Autodesk Inventor part; units mm, degrees
ref_plane "YZ Plane" through (0, 0, 0) normal (1, 0, 0) x (0, 1, 0)
ref_plane "XZ Plane" through (0, 0, 0) normal (0, 1, 0) x (-1, 0, 0)
ref_plane "XY Plane" through (0, 0, 0) normal (0, 0, 1) x (1, 0, 0)
sketch "Esboço9" plane through (0, 0, 0) normal (0, 0, 1) x (1, 0, 0)
  line L0 (-215, -43.375) -> (215, -43.375)
  line L1 (215, -43.375) -> (215, 42.625)
  line L2 (215, 42.625) -> (214.25, 42.625)
  line L3 (214.25, 42.625) -> (214.25, -42.625)
  line L4 (214.25, -42.625) -> (-214.25, -42.625)
  line L5 (-214.25, -42.625) -> (-214.25, 42.625)
  line L6 (-214.25, 42.625) -> (-215, 42.625)
  line L7 (-215, 42.625) -> (-215, -43.375)
  point P0 (0, 0)
  dimension "d60" = 430
  dimension "d61" = 86
  dimension "d64" = 85.25
  dimension "d65" = 428.5
  dimension "d67" = 0.75
  dimension "d107" = 214.25
  dimension "d109" = 42.625
extrude "Extrusão6" add sketch "Esboço9" against normal blind 180
sketch "Esboço10" plane through (-214.25, -42.625, 0) normal (0, 1, 0) x (1, 0, 0)
  line L0 (428.5, 0) -> (0, 0)
  line L1 (428.5, 0) -> (428.5, 0.75)
  line L2 (428.5, 0) -> (428.5, 180)
  line L3 (428.5, 0.75) -> (0, 0.75)
  line L4 (0, 0) -> (0, 180)
  line L5 (0, 180) -> (428.5, 180)
  line L6 (0, 180) -> (0, 179.25)
  line L7 (0, 0) -> (0, 180)
  line L8 (0, 179.25) -> (428.5, 179.25)
  line L9 (428.5, 179.25) -> (428.5, 180)
  line L10 (429.25, 180) -> (-0.75, 180)
  line L11 (0, 0.75) -> (0, 0)
  line L12 (-0.75, 0) -> (429.25, 0)
  line L13 (0, 180) -> (428.5, 180)
  point P0 (214.25, 0)
  dimension "d95" = 0.75
  dimension "d96" = 0.75
extrude "Extrusão7" add sketch "Esboço10" along normal blind 4.25 contours L0 L4 L3 L1 | L8 L4 L5 L2
sketch "Esboço11" plane through (214.25, 42.625, -180) normal (-1, 0, 0) x (0, 0, 1)
  line L0 (0, -81) -> (0.75, -81)
  line L1 (0.75, -81) -> (0, -81)
  line L2 (180, 0) -> (0, 0)
  line L3 (0, -81) -> (0, 0)
  line L4 (180, 0) -> (180, -81)
  line L5 (0, 0) -> (180, 0)
  line L6 (180, 0) -> (180, -81)
  line L7 (179.25, -81) -> (180, -81)
  line L8 (180, -81) -> (179.25, -81)
  line L9 (179.25, -81) -> (179.25, -0.75)
  line L10 (179.25, -0.75) -> (0.75, -0.75)
  line L11 (0.75, -0.75) -> (0.75, -81)
  point P0 (180, -42.625)
  dimension "d100" = 178.5
  dimension "d110" = 81
  dimension "d111" = 80.25
extrude "Extrusão8" add sketch "Esboço11" along normal blind 4.25
sketch "Esboço12" plane through (-214.25, 42.625, 0) normal (1, 0, 0) x (0, 0, -1)
  line L0 (0, -81) -> (0.75, -81)
  line L1 (0.75, -81) -> (0, -81)
  line L2 (0, -81) -> (0, 0)
  line L3 (180, -86) -> (180, 0)
  line L4 (0, 0) -> (180, 0)
  line L5 (179.25, -81) -> (180, -81)
  line L6 (180, 0) -> (180, -81)
  line L7 (180, -81) -> (179.25, -81)
  line L8 (179.25, -81) -> (179.25, -0.75)
  line L9 (179.25, -0.75) -> (0.75, -0.75)
  line L10 (0, -81) -> (0, 0)
  line L11 (0.75, -0.75) -> (0.75, -81)
  point P0 (0, -42.625)
  dimension "d103" = 80.25
  dimension "d104" = 178.5
  dimension "d112" = 81
extrude "Extrusão9" add sketch "Esboço12" along normal blind 4.25
sketch "Esboço15" plane through (-214.25, -42.625, -0.75) normal (0, 1, 0) x (1, 0, 0)
  circle A0 centre (311.2625, 145.825) radius 1.75
  circle A1 centre (288.7625, 89.075) radius 1.75
  line L0 (0, 0) -> (428.5, 0)
  line L1 (428.5, 0) -> (428.5, 178.5)
  line L2 (428.5, 178.5) -> (0, 178.5)
  line L3 (0, 0) -> (0, 178.5)
  circle A2 centre (260.7625, 89.075) radius 1.75
  circle A3 centre (238.2625, 145.825) radius 1.75
  circle A4 centre (192.2625, 145.825) radius 1.75
  circle A5 centre (169.7625, 89.075) radius 1.75
  circle A6 centre (141.7625, 89.075) radius 1.75
  circle A7 centre (119.2625, 145.825) radius 1.75
  circle A8 centre (91.2625, 145.825) radius 1.75
  circle A9 centre (68.7625, 89.075) radius 1.75
  circle A10 centre (40.7625, 89.075) radius 1.75
  circle A11 centre (18.2625, 145.825) radius 1.75
  circle A12 centre (339.2625, 145.825) radius 1.75
  circle A13 centre (389.7875, 89.3) radius 1.75
  circle A14 centre (412.2625, 145.825) radius 1.75
  circle A15 centre (361.7875, 89.3) radius 1.75
  point P0 (214.25, -0.75)
hole "Furo5" at (-195.9875, -42.625, -146.575) at (-122.9875, -42.625, -146.575) at (-145.4875, -42.625, -89.825) at (-173.4875, -42.625, -89.825) at (-94.9875, -42.625, -146.575) at (-72.4875, -42.625, -89.825) at (-44.4875, -42.625, -89.825) at (-21.9875, -42.625, -146.575) at (24.0125, -42.625, -146.575) at (46.5125, -42.625, -89.825) at (74.5125, -42.625, -89.825) at (97.0125, -42.625, -146.575) at (125.0125, -42.625, -146.575) at (198.0125, -42.625, -146.575) at (175.5375, -42.625, -90.05) at (147.5375, -42.625, -90.05) direction (0, -1, 0) diameter 2.459 end through all
properties part number "Ra-Manager_Base"
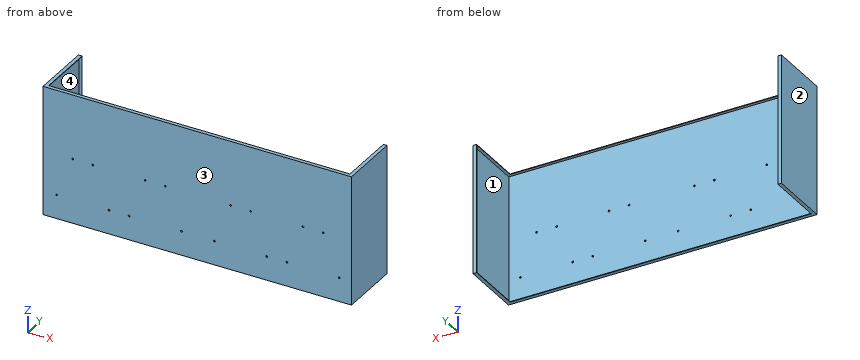
Work out the finished part from the listing and answer in its coordinate system (mm). Face numbers are marked on the shaded views. A direction names the side the tool comes from. Give positions to 0.01 mm unless a question says otherwise; leave off trailing zeros. Write each loop counter-clockwise with the first axis right and the second up, starting at its lowest first coordinate (ties: lowest second). Pieces come first, ordered by that corner, then holes.
(1) The mould has two halves that part along Z. Classify the marked faces 3 and 4: pulls with the +Z half, pulls with the -Z half, needs draft (parallel to the pull), parting line crosses it, or undercut.
Final values:
face 3: needs draft
face 4: undercut
(2) A flat-ended cylindrical pin translates along its axis: pin 1 Ø2 at (x, z) = (-10.5, -56.5) entering from +Y (3 decimals). Find the tip coordinate at first contact, or state that the pin passes through.
Final values:
pin 1: stops at y = -42.625
(3) The part is cut by section A-A on z = -47.5. Write down the section's boundary in (x, y) (3 decimals), plus the area to 3 significant figures.
Final values:
outline: (-215, -43.375) - (215, -43.375) - (215, 42.625) - (210, 42.625) - (210, 41.875) - (214.25, 41.875) - (214.25, -42.625) - (-214.25, -42.625) - (-214.25, 41.875) - (-210, 41.875) - (-210, 42.625) - (-215, 42.625) - close
area: 457 mm2
(4) Straight lines are drawn through the part: line 1 (X direction, y = 9.5, z = -108.5); line 2 (Y direction, x = 31, z = -51) (3 decimals). For each, find the intervals that lie inside material, in ascending order.
Final values:
line 1: x = -215 to -214.25, 214.25 to 215
line 2: y = -43.375 to -42.625
(5) Which of the six approach directions +Z, -Z, +X, -X, +Y, -Y give full straight-line access (tool end or side, diameter ignored) to the marked faces 1 and 2?
Final values:
face 1: none
face 2: +Z, -Z, -X, +Y, -Y
(6) The part is cut by section C-C on x = 52.5. Write down the section's boundary in (y, z) (3 decimals).
Final values:
outline: (-43.375, -180) - (-38.375, -180) - (-38.375, -179.25) - (-42.625, -179.25) - (-42.625, -0.75) - (-38.375, -0.75) - (-38.375, 0) - (-43.375, 0) - close
(7) The part is cut by section B-B on y = -3. Write down the section's boundary in (x, z), plus the area to 3 significant figures.
Final values:
outline: (-215, -180) - (-210, -180) - (-210, -179.25) - (-214.25, -179.25) - (-214.25, -0.75) - (-210, -0.75) - (-210, 0) - (-215, 0) - close; (210, -180) - (215, -180) - (215, 0) - (210, 0) - (210, -0.75) - (214.25, -0.75) - (214.25, -179.25) - (210, -179.25) - close
area: 283 mm2
